The model under review builds one solid part; all positions refer to its coordinate system, in mm. A direction names the side the tool comes from. Give positions to 0.01 mm unless a question says otherwise; leave off trailing zeros. Loops run counter-clockwise (first coordinate to the right, second up) from the corner with the lowest first, then second, coordinate; pieces in that order, holes last. Notation, with made-up numbers: M -39,57.5 L -5,57.5 A19 cw -5,71.5 Z; hole C 63,68.25 d7. An arc over 180 degrees is marked long. Put each result on its own line as item: value. Start each with the question number.
Autodesk Inventor part; units mm, degrees
ref_plane "YZ Plane" through (0, 0, 0) normal (1, 0, 0) x (0, 1, 0)
ref_plane "XZ Plane" through (0, 0, 0) normal (0, 1, 0) x (-1, 0, 0)
ref_plane "XY Plane" through (0, 0, 0) normal (0, 0, 1) x (1, 0, 0)
sketch "Sketch1" plane through (0, 0, 0) normal (0, 1, 0) x (-1, 0, 0)
  line L0 (-5.5, -3) -> (-11.5, -3)
  line L1 (-11.5, -3) -> (-11.5, 3)
  line L2 (-11.5, 3) -> (-5.5, 3)
  line L3 (-5.5, 3) -> (-5.5, -3)
  line L4 (-5.5, -3) -> (-11.5, 3) construction
  line L5 (-11.5, -3) -> (-5.5, 3) construction
  line L6 (11.5, -3) -> (5.5, -3)
  line L7 (5.5, -3) -> (5.5, 3)
  line L8 (5.5, 3) -> (11.5, 3)
  line L9 (11.5, 3) -> (11.5, -3)
  line L10 (11.5, -3) -> (5.5, 3) construction
  line L11 (5.5, -3) -> (11.5, 3) construction
  point P0 (0, 0)
  point P1 (-8.5, 0)
  point P2 (8.5, 0)
  dimension "d0" = 6
  dimension "d1" = 6
  dimension "d2" = 0
  dimension "d3" = 5.5
  dimension "d4" = 6
  dimension "d5" = 6
  dimension "d7" = 11
extrude "Extrusion1" add sketch "Sketch1" against normal blind 1
sketch "Sketch2" plane through (0, -1, 0) normal (0, -1, 0) x (1, 0, 0)
  line L0 (-5.5, 3) -> (-11.5, 3)
  line L1 (-5.5, 3) -> (-5.5, -3)
  line L2 (-11.5, 3) -> (-5.5, 3)
  line L3 (-5.5, 3) -> (-5.5, 1)
  line L4 (-5.5, 1) -> (-11.5, 1)
  line L5 (-11.5, 1) -> (-11.5, 3)
  line L6 (-5.5, -3) -> (-11.5, -3)
  line L7 (-11.5, -3) -> (-5.5, -3)
  line L8 (-5.5, -3) -> (-5.5, -1)
  line L9 (-5.5, -1) -> (-11.5, -1)
  line L10 (-11.5, -1) -> (-11.5, -3)
  line L11 (5.5, 3) -> (5.5, -3)
  line L12 (11.5, -3) -> (11.5, 3)
  line L13 (5.5, 3) -> (11.5, 3)
  line L14 (11.5, 3) -> (11.5, 1)
  line L15 (11.5, 1) -> (5.5, 1)
  line L16 (5.5, 1) -> (5.5, 3)
  line L17 (5.5, -3) -> (11.5, -3)
  line L18 (5.5, -3) -> (11.5, -3)
  line L19 (11.5, -3) -> (11.5, -1)
  line L20 (11.5, -1) -> (5.5, -1)
  line L21 (5.5, -1) -> (5.5, -3)
  point P0 (0, 0)
  dimension "d10" = 2
  dimension "d11" = 2
extrude "Extrusion2" add sketch "Sketch2" along normal blind 6 contours L1 L4 L5 L0 | L1 L6 L10 L9 | L13 L12 L15 L11 | L20 L12 L17 L11
sketch "Sketch3" plane through (0, 0, 0) normal (0, 1, 0) x (1, 0, 0)
  line L0 (-11.5, 1) -> (-11.5, 3)
  line L1 (-11.5, 1) -> (11.5, 1)
  line L2 (11.5, 1) -> (11.5, 19)
  line L3 (11.5, 19) -> (-11.5, 19)
  line L4 (-11.5, 19) -> (-11.5, 1)
  line L5 (-5.5, 3) -> (-11.5, 3)
  circle A0 centre (-9.5, 17) radius 1
  circle A1 centre (-9.5, 5) radius 1
  point P0 (0, 0)
  dimension "d14" = 23
  dimension "d15" = 16
  dimension "d16" = 2
  dimension "d17" = 2
  dimension "d18" = 2
  dimension "d19" = 2
  dimension "d20" = 2
  dimension "d21" = 2
extrude "Extrusion3" add sketch "Sketch3" against normal blind 2
fillet "Fillet1" radius 2 2 edges at (-8.5, -2, -3) (8.5, -2, -3)
properties part number "sensor_3DPrint"
Item 1: Consider section D-D, the plane z = -0.25. Write out the cut boundary in (x, y).
Item 2: Tool access review of faces 1 (the flat face through (0, -2, -10)), 2 (the flat face through (9, -1, 0)), 3 (the flat face through (-5.5, -4, -2)), 4 (the flat face through (0, 0, -8)), 5 (the flat face through (-9, -5, -3)): name each direction out of +Z, -Z, +X, -X, +Y, -Y from which nothing blocks a thin tool from reaching the whole face with its end or side.
Item 3: Draft analysis for pull direction X (two halves, no side actions). For faces 6 (the cylindrical face through (-9.717, -1.118, -4.024)), 7 (the flat face through (8, -7, -2)), 8 (the flat face through (5.5, -3, 2)), 9 (the flat face through (-11.5, -1, -5)), state which applies: +X half, -X half, draft (parallel to the pull), parting line (faces both ways), or undercut.
Item 4: To check wall thickness, follow L1, parallel to Z at x = -9.5, y = -0.75; L2, parallel to X at y = -0.9, z = -5; L3, parallel to X at y = -2.25, z = -2. State the ranges of each line that lie inside material, in increasing order. Write a range as [from, to].
Item 5: Consider section C-C, the plane y = -5.75. Write out the cut boundary in (x, z), plus the area to 3 significant figures.
Item 6: Clearance check with flat-ended pins moving along their axes: pin 1 Ø3 at (x, y) = (-7.5, -5) entering from -Z; pin 2 Ø1.2 at (x, z) = (-9.5, -5) entering from +Y; pin 3 Ø2 at (x, y) = (-7.5, -6) entering from -Z; pin 4 Ø4 at (y, z) = (-5, 0) entering from -X. State where each tip first meets the part, or that it passes through.
Item 7: Consider section A-A, the plane z = -17. Write out the cut boundary in (x, y).
Item 8: Consider section B-B, the plane x = -9.5. Write out the cut boundary in (y, z).
Report:
1. outline: M -11.5,-1 L -5.5,-1 L -5.5,0 L -11.5,0 Z; M 5.5,-1 L 11.5,-1 L 11.5,0 L 5.5,0 Z
2. face 1: -Z, -Y
2. face 2: +X, -X, -Y
2. face 3: +Z, -Z, -Y
2. face 4: +Z, -Z, +X, -X, +Y
2. face 5: -Z, +X, -X, -Y
3. face 6: undercut
3. face 7: draft
3. face 8: undercut
3. face 9: -X half
4. L1: [-19, -18], [-16, -6], [-4, 3]
4. L2: [-11.5, -10.5], [-8.5, 11.5]
4. L3: [-11.5, -5.5], [5.5, 11.5]
5. outline: M -11.5,-3 L -5.5,-3 L -5.5,-1 L -11.5,-1 Z; M -11.5,1 L -5.5,1 L -5.5,3 L -11.5,3 Z; M 5.5,-3 L 11.5,-3 L 11.5,-1 L 5.5,-1 Z; M 5.5,1 L 11.5,1 L 11.5,3 L 5.5,3 Z
5. area: 48.0 mm²
6. pin 1: z = -3.06
6. pin 2: through
6. pin 3: z = -3
6. pin 4: x = -11.5
7. outline: M -11.5,-2 L -10.5,-2 L -10.5,0 L -11.5,0 Z; M -8.5,-2 L 11.5,-2 L 11.5,0 L -8.5,0 Z
8. outline: M -7,-3 L -4,-3 A2 cw -2.27,-4 L 0,-4 L 0,3 L -7,3 L -7,1 L -1,1 L -1,-1 L -7,-1 Z; M -2,-19 L 0,-19 L 0,-18 L -2,-18 Z; M -2,-16 L 0,-16 L 0,-6 L -2,-6 Z
